Verification items for the finished model (mm, model axes). Face numbers are marked on the shaded views. Coordinates: 2 decimals unless noted, no trailing zeros. Order: outer loops, then holes, each group sorted by start corner. A loop starts at its lowest first (then second) coordinate and runs counter-clockwise, first axis right, second up. Notation, with made-up numbers: (-13, -27.75) - (-7, -27.75) arc R28 ccw to (-7, 2.25) - close; hole circle Ø11 at (-37, -34.5). An arc over 180 degrees is marked (long way). One line per question, with ' | ' between items. Start each with the question number.
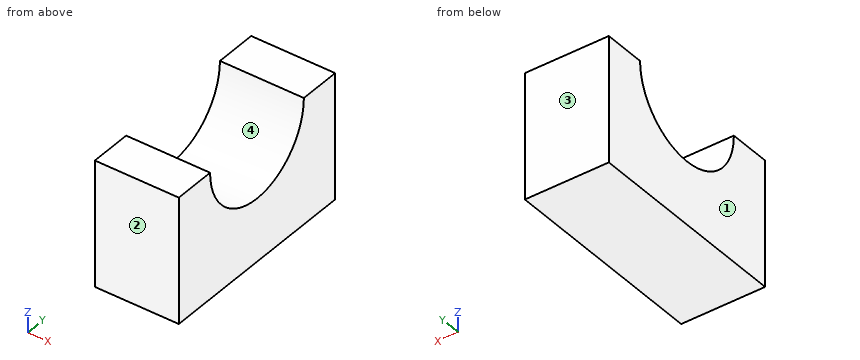
from build123d import *

# Parameters (mm, degrees)
F0_W     = 25.4
F0_H     = 38.1
F1_DEPTH = 63.5
F3_DEPTH = 25.4


with BuildPart() as f1:
    # F0 (on Front) → F1 (new body)
    with BuildSketch(Plane.XZ):
        with Locations((12.7, 19.05)):
            Rectangle(F0_W, F0_H)
    extrude(amount=F1_DEPTH)

    # F2 (on face) → F3 (cut)
    with BuildSketch(Plane.YZ.offset(25.4)):
        with BuildLine():
            ThreePointArc((-50.8, 38.1), (-31.75, 19.05), (-12.7, 38.1))
            Line((-12.7, 38.1), (-50.8, 38.1))
        make_face()
    extrude(amount=-F3_DEPTH, mode=Mode.SUBTRACT)


solid = f1.part
Item 1: Mould release check, pull along Y, two halves, no side actions. Record for the marked faces 1, 2, 3 and 4: +Y half, -Y half, draft (parallel to the pull), parting line (faces both ways), or undercut.
Item 2: Gauge pin test, flat ends, axial feed: pin 1 (12 mm diameter, centred on x = 12.5, y = -40.5, fed in from +Z); pin 2 (4 mm diameter, centred on x = 8.5, y = -24.5, fed in from +Z). Record the tip position at first contact, or that the pin passes through.
Item 3: Section check D-D (y = -19.5). Record the cut outline in (x, z), then the cut area to 3 significant figures.
Item 4: Thickness scan on probe 1 along Y at (x, z) = (15.5, 30.5); probe 2 along Y at (x, z) = (10.25, 31); probe 3 along Z at (x, y) = (6, -27). Record the ranges inside material, lowest first. Write a range as from..to.
Item 5: Section check A-A (z = 36). Record the cut outline in (x, y).
Item 6: Section check C-C (y = -31.75). Record the cut outline in (x, z), then the cut area to 3 significant figures.
Item 7: Section check B-B (x = 1.75). Record the cut outline in (y, z), then the cut area to 3 significant figures.
Completed:
1) face 1: draft | face 2: -Y half | face 3: +Y half | face 4: undercut
2) pin 1: stops at z = 26.04 | pin 2: stops at z = 21.45
3) outline: (0, 0) - (25.4, 0) - (25.4, 23.51) - (0, 23.51) - close | area: 597 mm^2
4) probe 1: y = -63.5..-49.22, -14.28..0 | probe 2: y = -63.5..-49.43, -14.07..0 | probe 3: z = 0..19.65
5) outline: (0, -63.5) - (25.4, -63.5) - (25.4, -50.68) - (0, -50.68) - close; (0, -12.82) - (25.4, -12.82) - (25.4, 0) - (0, 0) - close
6) outline: (0, 0) - (25.4, 0) - (25.4, 19.05) - (0, 19.05) - close | area: 484 mm^2
7) outline: (-63.5, 0) - (0, 0) - (0, 38.1) - (-12.7, 38.1) arc R19.05 cw to (-50.8, 38.1) - (-63.5, 38.1) - close | area: 1,850 mm^2
